For this review, take the finished solid that the model builds, in its own axes (mm). A direction names the side the tool comes from. Give positions to 0.01 mm unless a question says otherwise; leave off trailing zeros. Order: outer loops, then holes, each group sorted by start corner. A loop starts at its lowest first (then second) coordinate and runs counter-clockwise, first axis right, second up. Notation, with made-up numbers: (-38.5, 45.25) - (10.5, 45.25) arc R20 ccw to (10.5, 56.25) - close; hole circle Ø7 at (65.25, 46.25). An arc over 180 degrees is marked (long way). Use a Markdown table: item, result. Add a question column.
1) Clearance check with flat-ended pins moving along their axes: P1, Ø10, axis at y = -21, z = 5, coming from the -X side; P2, Ø19.5, axis at x = 37.5, z = 16, coming from the +Y side; P3, Ø7, axis at y = -2, z = 10.5, coming from the -X side. State where each tip first meets the part, or that it passes through.
2) We need section B-B on x = 14.5. Write out the cut boundary in (y, z).
3) We need section A-A on z = 19.05. Write out the cut boundary in (x, y).
4) We need section C-C on z = 27. Write out the cut boundary in (x, y).
5) Wall thickness on L1, parallel to Z at x = 24.5, y = -1.5; L2, parallel to Y at x = 36, z = 28.5: over which ranges is each line inside the solid? List them lowest first.
6) We need section D-D on y = -53. Write out the cut boundary in (x, z).
7) Machinability: for faces 1 (the face through (34, -6.35, 19)), 2 (the face through (57.13, -87.96, 18.78)), 3 (the face through (43, -95.25, 19)), 4 (the face through (0, -3, 19)), which of the approach directions +Z, -Z, +X, -X, +Y, -Y give a long, thin tool a straight path to every point of the face, cutting with its end or side? Answer none if there is none.
8) Mouldability with a two-part tool opening along Z and no side actions: class faces 5 (the face through (30.557, -3.131, 17.143)), 6 (the face through (58.051, -48, 19)), 7 (the face through (61, -47, 0)), 8 (the face through (61, -47, 38.1)) as released by +Z, released by -Z, zero draft, split by the parting line, or undercut.
```python
from build123d import *

# Parameters (mm, degrees)
BOSS_EXTRUDE1_DEPTH = 38.1
SKETCH2_R           = 6.35
CUT_EXTRUDE1_DEPTH  = 38.1


with BuildPart() as part:
    # Sketch1 → Boss-Extrude1 (new body)
    with BuildSketch(Plane.XY):
        with BuildLine():
            Line((0, 0), (53.98, 0))
            ThreePointArc((53.98, 0), (61.287211447, -2.441393787), (64.401363743, -9.488222735))
            Line((64.401363743, -9.488222735), (64.401363743, -85.721240556))
            ThreePointArc((64.401363743, -85.721240556), (61.664237719, -92.40538322), (55.025128035, -95.25))
            Line((55.025128035, -95.25), (30.071323434, -95.25))
            ThreePointArc((30.071323434, -95.25), (27.161692752, -94.580250085), (24.602099349, -93.043045718))
            Line((24.602099349, -93.043045718), (-7.280670374, -66.290225402))
            Line((-7.280670374, -66.290225402), (-3.198969052, -61.425843189))
            Line((-3.198969052, -61.425843189), (28.68380067, -88.178663504))
            ThreePointArc((28.68380067, -88.178663504), (29.463882201, -88.660646082), (30.349062467, -88.9))
            Line((30.349062467, -88.9), (54.96018039, -88.9))
            ThreePointArc((54.96018039, -88.9), (57.151148485, -87.938216318), (58.051363743, -85.721240556))
            Line((58.051363743, -85.721240556), (58.051363743, -9.488222735))
            ThreePointArc((58.051363743, -9.488222735), (56.930321756, -7.064776449), (54.357595252, -6.35))
            Line((54.357595252, -6.35), (0, -6.35))
            Line((0, -6.35), (0, 0))
        make_face()
    extrude(amount=BOSS_EXTRUDE1_DEPTH)

    # Sketch2 → Cut-Extrude1 (cut)
    with BuildSketch(Plane(origin=(0, 0, 0), x_dir=(1, 0, 0), z_dir=(0, 1, 0))):
        with Locations((24.5, -19.05)):
            Circle(SKETCH2_R)
    extrude(amount=-CUT_EXTRUDE1_DEPTH, mode=Mode.SUBTRACT)


solid = part.part
```
Checked values:
| question | item | result |
|---|---|---|
| 1 | P1 | x = 58.05 |
| 1 | P2 | y = 0 |
| 1 | P3 | x = 0 |
| 2 | outline | (-84.57, 0) - (-76.28, 0) - (-76.28, 38.1) - (-84.57, 38.1) - close; (-6.35, 0) - (0, 0) - (0, 38.1) - (-6.35, 38.1) - close |
| 3 | outline | (-7.28, -66.29) - (24.6, -93.04) arc R9.53 ccw to (30.07, -95.25) - (55.03, -95.25) arc R9.53 ccw to (64.4, -85.72) - (64.4, -9.49) arc R9.53 ccw to (53.98, 0) - (30.85, 0) - (30.85, -6.35) - (54.36, -6.35) arc R3.18 cw to (58.05, -9.49) - (58.05, -85.72) arc R3.18 cw to (54.96, -88.9) - (30.35, -88.9) arc R3.18 cw to (28.68, -88.18) - (-3.2, -61.43) - close; (0, -6.35) - (18.15, -6.35) - (18.15, 0) - (0, 0) - close |
| 4 | outline | (-7.28, -66.29) - (24.6, -93.04) arc R9.53 ccw to (30.07, -95.25) - (55.03, -95.25) arc R9.53 ccw to (64.4, -85.72) - (64.4, -9.49) arc R9.53 ccw to (53.98, 0) - (0, 0) - (0, -6.35) - (54.36, -6.35) arc R3.18 cw to (58.05, -9.49) - (58.05, -85.72) arc R3.18 cw to (54.96, -88.9) - (30.35, -88.9) arc R3.18 cw to (28.68, -88.18) - (-3.2, -61.43) - close |
| 5 | L1 | 0 to 12.7, 25.4 to 38.1 |
| 5 | L2 | -95.25 to -88.9, -6.35 to 0 |
| 6 | outline | (58.05, 0) - (64.4, 0) - (64.4, 38.1) - (58.05, 38.1) - close |
| 7 | face 1 | +Z, -Z, -X |
| 7 | face 2 | +Z, -Z |
| 7 | face 3 | +Z, -Z, +X, -X, -Y |
| 7 | face 4 | +Z, -Z, -X, +Y |
| 8 | face 5 | undercut |
| 8 | face 6 | zero draft |
| 8 | face 7 | released by -Z |
| 8 | face 8 | released by +Z |
